Verification items for the finished model (mm, model axes). A direction names the side the tool comes from. Round coordinates to 2 decimals unless told otherwise and drop trailing zeros. Write each loop counter-clockwise with the first axis right and the second up, starting at its lowest first coordinate (ties: lowest second). Pieces come first, ordered by that corner, then holes. Notation, with made-up numbers: M 31,-22.5 L 78,-22.5 A10 ccw 78,-18.5 Z; hole C 71.25,69 d4. An arc over 180 degrees is marked long. One line per question, with ' | ' between items. Start each with the question number.
Q1. Release check for a two-part mould opening along Z. For faces 1 (the face through (8, 1, 0)), 2 (the face through (7, -0.75, 0)), 3 (the face through (3.84, -1.5, -0.07)) record: released by +Z, released by -Z, zero draft, split by the parting line, or undercut.
Q2. Gauge pin test, flat end, axial feed: pin 1 (1.5 mm diameter, centred on x = 2, y = 1, fed in from +Z). Record the tip position at first contact, or that the pin passes through.
Q3. Tool access check on faces 4 (the face through (7, 0.75, 0)), 5 (the face through (0, 0, 0)). Record the directions out of +Z, -Z, +X, -X, +Y, -Y that give a thin tool (end or side, any length) a straight path to the whole face; none if there is none.
Q4. Cross-section at A-A (x = 1.25). Record the boundary of the cut face in (y, z).
Q5. Thickness scan on line 1 along Z through (x, y) = (4.75, 1.3); line 2 along X through (y, z) = (0.05, 0.05); line 3 along X through (y, z) = (-0.6, -0.9). Record the ranges inside material, lowest first. Write a range as from..to.
Autodesk Inventor part; units mm, degrees
ref_plane "Work Plane1" through (4, 0, 0) normal (0, 0.5, 0.866) x (1, 0, 0)
ref_plane "YZ Plane" through (0, 0, 0) normal (1, 0, 0) x (0, 1, 0)
ref_plane "XZ Plane" through (0, 0, 0) normal (0, 1, 0) x (-1, 0, 0)
sketch "Sketch1" plane through (0, 0, 0) normal (0, 0, 1) x (1, 0, 0)
  line L0 (0, 0) -> (6.3, 0)
  line L1 (8, 0.866) -> (8, 1.5)
  line L2 (8, 1.5) -> (0, 1.5)
  line L3 (8, 0.866) -> (6.8, 0.866)
  line L4 (6.8, 0.866) -> (6.3, 0)
  line L5 (0, -0.3) -> (0, 1.8)
  line L6 (0, 1.5) -> (0, 0)
  dimension "d0" = 1.2
  dimension "d1" = 60
  dimension "d2" = 3
  dimension "d3" = 1.7321
  dimension "d5" = 8
revolve "Body" add sketch "Sketch1" angle 360 about axis through (0, 0, 0) along (1, 0, 0)
chamfer "Chamfer1" distance 0.3067 angle 60 1 edges at (8, -1.5, 0) measured on face at (8, 1.2658, -0.1887)
sketch "Sketch2" plane through (8, 0, 0) normal (1, 0, 0) x (0, 0, -1)
  circle A0 centre (0, 0) radius 0.866
  line L0 (-0.433, 0.75) -> (0.433, 0.75)
  line L1 (0.433, 0.75) -> (0.866, 0)
  line L2 (0.866, 0) -> (0.433, -0.75)
  line L3 (0.433, -0.75) -> (-0.433, -0.75)
  line L4 (-0.433, -0.75) -> (-0.866, 0)
  line L5 (-0.866, 0) -> (-0.433, 0.75)
extrude "Slot" add sketch "Sketch2" against normal up to next contours L1 A0 | A0 L2 | L0 A0 | A0 L3 | L5 A0 | A0 L4
thread "Thread"
chamfer "Chamfer2" distance 0.3067 angle 60 1 edges at (0, -1.5, 0) measured on face at (2.4896, 1.4806, -0.2406)
ref_plane "Work Plane1" through (4, 0, 0) normal (0, 0.5, 0.866) x (1, 0, 0)
equation "\"d0\" = INTI"
equation "\"d2\" = NND"
equation "\"d3\" = 1.1547 * SW"
equation "\"d7\" = -0.5 * GD1 + 0.5 * NND"
equation "\"d8\" = FAWI"
equation "\"d29\" = -0.5 * GD1 + 0.5 * NND"
equation "\"d13\" = -0.5 * GD1 + 0.5 * NND"
equation "\"d14\" = FAWI"
equation "\"d30\" = -0.5 * GD1 + 0.5 * NND"
equation "\"NND\" = 3"
equation "\"NLG\" = 3"
equation "\"INTI\" = 1.2"
equation "\"FAWI\" = 60deg"
equation "\"SW\" = 1.5"
equation "\"GD1\" = THREADDIA - 1.2269 * PTC"
equation "\"FAWI1\" = 45deg"
equation "\"GUL\" = 0.61345 * PTC"
equation "\"SPD\" = 2"
equation "\"SEWI\" = 120deg"
equation "\"TOA\" = 30deg"
equation "\"THREADDIA\" = 3"
equation "\"PTC\" = 0.5"
equation "\"GAL\" = 0.61345 * PTC"
equation "\"E0\" = 1.155 * SW"
properties part number "Grub Screw 3x8mm" material "Stainless Steel, 440C"
Determined:
1) face 1: zero draft | face 2: undercut | face 3: split by the parting line
2) pin 1: stops at z = 1.48
3) face 4: +X | face 5: +Z, -Z, -X, +Y, -Y
4) outline: C 0,0 d3
5) line 1: z = -0.75..0.75 | line 2: x = 0..6.34 | line 3: x = 0.07..8
